Design review of the part built by this model. Coordinates are the model's own, in mm. Face numbers are marked on the shaded views. A direction names the side the tool comes from. Coordinates: 2 decimals unless noted, no trailing zeros. Write each loop counter-clockwise with the first axis right and the second up, starting at its lowest first coordinate (ties: lowest second). Pieces come first, ordered by that corner, then holes.
Q1. The part is to be moulded in two halves that separate along Z. For the marked faces 1, 2 and 3, say which applies: released by +Z, released by -Z, zero draft, split by the parting line, or undercut.
Q2. Take a section at B-B, the plane x = 0. Write out the cut boundary in (y, z), plus the area to 3 significant figures.
Q3. Take a section at C-C, the plane y = -12.5. Write out the cut boundary in (x, z), plus the area to 3 significant figures.
Q4. Take a section at D-D, the plane x = 1.75. Write out the cut boundary in (y, z), plus the area to 3 significant figures.
Q5. Take a section at A-A, the plane y = 7.75. Write out the cut boundary in (x, z).
Q6. For pin 1 Ø5 at (y, z) = (-4, -2) entering from +X; pin 2 Ø2.5 at (x, y) = (-0.5, 6.5) entering from -Z; pin 3 Ø3 at (x, y) = (-0.5, 7) entering from +Z; pin 4 Ø5 at (y, z) = (-5, -3.5) entering from -X, all flat-tipped, find the tip position at first contact; note any pin that passes through.
Q7. For the marked faces 4, 5 and 6, list the 3-axis set-ups (+Z, -Z, +X, -X, +Y, -Y) from which the entire face can be reached by the end or side of a thin tool; tool diameter is ignored.
Q8. For L1, parallel to Y at x = 1.85, z = 0; L2, parallel to Z at x = -0.25, y = 6.5; L3, parallel to X at y = 9.5, z = -0.5, list the stretches that pass through material, from the lowest coordinate up.
from build123d import *

# Parameters (mm, degrees)
BOSS_EXTRUDE1_DEPTH              = 5
BOSS_EXTRUDE1_DEPTH_BACK         = 5
SKETCH1_R                        = 5
SKETCH2_W                        = 5
SKETCH2_H                        = 8.660254038
BOSS_EXTRUDE2_DEPTH              = 10
CUT_EXTRUDE1_DEPTH               = 10
F_95_0_03937008_DIAMETER_HOLE1_D = 1.000000032
CUT_EXTRUDE2_DEPTH               = 10
CUT_EXTRUDE2_DEPTH_BACK          = 22.213203436
SKETCH7_W                        = 2.5
SKETCH7_H                        = 2.5
SKETCH8_W                        = 5
SKETCH8_H                        = 8.660254038
BOSS_EXTRUDE3_DEPTH              = 7.5
CUT_EXTRUDE3_DEPTH               = 7.5
F_95_0_03937008_DIAMETER_HOLE2_D = 1.000000032
SKETCH13_W                       = 2.5
SKETCH13_H                       = 2.5
CUT_EXTRUDE4_DEPTH               = 7.5


with BuildPart() as part:
    # Sketch1 → Boss-Extrude1 (new, two sides: drawn at the far end of the back side and taken through both)
    with BuildSketch(Plane(origin=(0, 0, 0), x_dir=(1, 0, 0), z_dir=(0, 1, 0)).offset(-BOSS_EXTRUDE1_DEPTH_BACK)):
        with Locations(Location((0, 0, 0), (0, 0, 270))):
            Circle(SKETCH1_R)
    extrude(amount=BOSS_EXTRUDE1_DEPTH + BOSS_EXTRUDE1_DEPTH_BACK)

    # Sketch2 → Boss-Extrude2 (add)
    with BuildSketch(Plane(origin=(0, -5, 0), x_dir=(-1, 0, 0), z_dir=(0, -1, 0))):
        Rectangle(SKETCH2_W, SKETCH2_H)
    extrude(amount=BOSS_EXTRUDE2_DEPTH)

    # Sketch3 → Cut-Extrude1 (cut)
    with BuildSketch(Plane.ZY.offset(2.5)):
        with BuildLine():
            Line((4.330127019, -10.66987298), (5.842852499, -10.66987298))
            Line((5.842852499, -10.66987298), (5.842852499, -18.914150706))
            Line((5.842852499, -18.914150706), (-6.856243272, -18.914150706))
            Line((-6.856243272, -18.914150706), (-6.856243272, -10.66987298))
            Line((-6.856243272, -10.66987298), (-4.330127019, -10.66987298))
            ThreePointArc((-4.330127019, -10.66987298), (-3.061862179, -13.731735159), (0, -15))
            ThreePointArc((0, -15), (3.061862179, -13.731735159), (4.330127019, -10.66987298))
        make_face()
    extrude(amount=-CUT_EXTRUDE1_DEPTH, mode=Mode.SUBTRACT)

    # 95 _0.03937008_ Diameter Hole1 (through all)
    with Locations(Plane.ZY.offset(2.5)):
        with Locations((0, -12.499999999)):
            Hole(F_95_0_03937008_DIAMETER_HOLE1_D / 2)

    # Sketch7 → Cut-Extrude2 (cut, two sides: drawn at the far end of the back side and taken through both)
    with BuildSketch(Plane(origin=(0, 5, 0), x_dir=(1, 0, 0), z_dir=(0, 1, 0)).offset(-CUT_EXTRUDE2_DEPTH_BACK)):
        Rectangle(SKETCH7_W, SKETCH7_H)
    extrude(amount=CUT_EXTRUDE2_DEPTH + CUT_EXTRUDE2_DEPTH_BACK, mode=Mode.SUBTRACT)

    # Sketch8 → Boss-Extrude3 (add)
    with BuildSketch(Plane(origin=(0, 5, 0), x_dir=(1, 0, 0), z_dir=(0, 1, 0))):
        Rectangle(SKETCH8_W, SKETCH8_H)
    extrude(amount=BOSS_EXTRUDE3_DEPTH)

    # Sketch9 → Cut-Extrude3 (cut)
    with BuildSketch(Plane.ZY.offset(2.5)):
        with BuildLine():
            Line((-4.330127019, 8.16987298), (-5.309333273, 8.16987298))
            Line((-5.309333273, 8.16987298), (-5.309333273, 13.114789022))
            Line((-5.309333273, 13.114789022), (5.138804432, 13.114789022))
            Line((5.138804432, 13.114789022), (5.138804432, 8.16987298))
            Line((5.138804432, 8.16987298), (4.330127019, 8.16987298))
            ThreePointArc((4.330127019, 8.16987298), (0, 12.499999999), (-4.330127019, 8.16987298))
        make_face()
    extrude(amount=-CUT_EXTRUDE3_DEPTH, mode=Mode.SUBTRACT)

    # 95 _0.03937008_ Diameter Hole2 (through all)
    with Locations(Plane.ZY.offset(2.5)):
        with Locations((0, 9.999999999)):
            Hole(F_95_0_03937008_DIAMETER_HOLE2_D / 2)

    # Sketch13 → Cut-Extrude4 (cut)
    with BuildSketch(Plane.XZ.offset(-5)):
        Rectangle(SKETCH13_W, SKETCH13_H)
    extrude(amount=-CUT_EXTRUDE4_DEPTH, mode=Mode.SUBTRACT)


solid = part.part
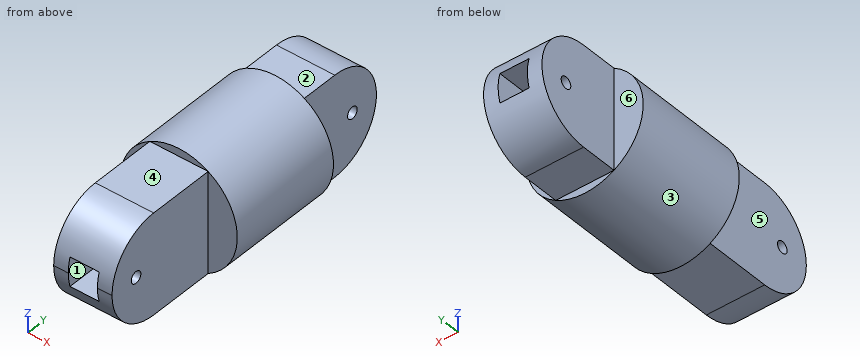
Responses:
1. face 1: undercut
1. face 2: released by +Z
1. face 3: split by the parting line
2. outline: (-14.82, -1.25) arc R4.33 ccw to (-10.67, -4.33) - (-5, -4.33) - (-5, -5) - (5, -5) - (5, -4.33) - (8.17, -4.33) arc R4.33 ccw to (12.32, -1.25) - close; (-14.82, 1.25) - (12.32, 1.25) arc R4.33 ccw to (8.17, 4.33) - (5, 4.33) - (5, 5) - (-5, 5) - (-5, 4.33) - (-10.67, 4.33) arc R4.33 ccw to start
2. area: 167 mm2
3. outline: (-2.5, -3.92) - (2.5, -3.92) - (2.5, -0.5) - (1.25, -0.5) - (1.25, -1.25) - (-1.25, -1.25) - (-1.25, -0.5) - (-2.5, -0.5) - close; (-2.5, 0.5) - (-1.25, 0.5) - (-1.25, 1.25) - (1.25, 1.25) - (1.25, 0.5) - (2.5, 0.5) - (2.5, 3.92) - (-2.5, 3.92) - close
3. area: 30.5 mm2
4. outline: (-10.67, -4.33) - (-5, -4.33) - (-5, -4.68) - (5, -4.68) - (5, -4.33) - (8.17, -4.33) arc R4.33 ccw to (8.17, 4.33) - (5, 4.33) - (5, 4.68) - (-5, 4.68) - (-5, 4.33) - (-10.67, 4.33) arc R4.33 ccw to start; hole circle Ø1 at (-12.5, 0); hole circle Ø1 at (10, 0)
4. area: 228 mm2
5. outline: (-2.5, -4.33) - (2.5, -4.33) - (2.5, 4.33) - (-2.5, 4.33) - close; hole (-1.25, -1.25) - (1.25, -1.25) - (1.25, 1.25) - (-1.25, 1.25) - close
6. pin 1: stops at x = 5
6. pin 2: stops at z = -4.33
6. pin 3: stops at z = 4.33
6. pin 4: stops at x = -4.9
7. face 4: +Z, +X, -X, -Y
7. face 5: +Z, -Z, -X, -Y
7. face 6: +Z, -Z, -X, +Y
8. L1: y = -15 to -13, -12 to 9.5, 10.5 to 12.5
8. L2: z = -4.33 to -1.25, 1.25 to 4.33
8. L3: x = -2.5 to -1.25, 1.25 to 2.5
